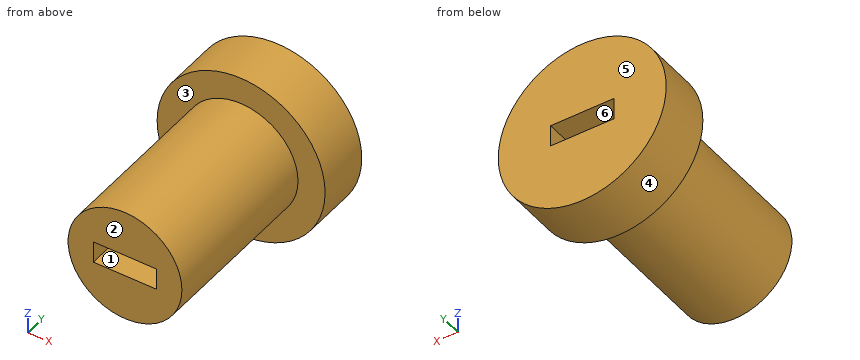
from build123d import *

# Parameters (mm, degrees)
F0_R     = 4.65
F0_R_2   = 3.15
F0_W     = 3.5
F0_H     = 1.2
F1_DEPTH = 2
F2_DEPTH = 3
F3_DEPTH = 12.5


with BuildPart() as f1:
    # F0 (on Front) → F1 (new body)
    with BuildSketch(Plane.XZ):
        Circle(F0_R)
        Circle(F0_R_2, mode=Mode.SUBTRACT)
        Circle(F0_R_2)
        Rectangle(F0_W, F0_H, mode=Mode.SUBTRACT)
    extrude(amount=F1_DEPTH)

    # F0 (on Front) → F2 (join)
    with BuildSketch(Plane.XZ):
        Circle(F0_R)
        Circle(F0_R_2, mode=Mode.SUBTRACT)
        Circle(F0_R_2)
        Rectangle(F0_W, F0_H, mode=Mode.SUBTRACT)
    extrude(amount=F2_DEPTH)

    # F0 (on Front) → F3 (join)
    with BuildSketch(Plane.XZ):
        Circle(F0_R_2)
        Rectangle(F0_W, F0_H, mode=Mode.SUBTRACT)
    extrude(amount=F3_DEPTH)


solid = f1.part
Here's how the part is built. I have some questions about the finished solid (model axes, mm). Face numbers are marked on the shaded views. A direction names the side the tool comes from. Coordinates: 2 decimals unless noted, no trailing zeros. Order: outer loops, then holes, each group sorted by start corner. A loop starts at its lowest first (then second) coordinate and runs counter-clockwise, first axis right, second up. Notation, with made-up numbers: (-3.5, -33.75) - (55.5, -33.75) arc R19 cw to (55.5, -18.75) - close; hole circle Ø1 at (31, 58). An arc over 180 degrees is marked (long way). Use CSV: the item, a comma, the result in double quotes. Start each with the question number.
1. Please list where these lines run through material, in increasing order: line 1 (Z direction, x = 0, y = -7.75); line 2 (X direction, y = -6, z = -0.5); line 3 (Z direction, x = -1.5, y = -2.75). Write a range as from..to.
2. For the marked faces 1, 2 and 3, which set-ups out of +Z, -Z, +X, -X, +Y, -Y let a thin tool reach every point of the face, with its end or its side?
3. If we mould it in two halves opening along X, with no side actions, what happens to the marked faces 4, 5 and 6? For each: +X half, -X half, draft (parallel to the pull), parting line (faces both ways), or undercut.
4. Suppose I cut it at D-D on z = -1. List the corners of the cut face in (x, y) for me, then the cut area to 3 significant figures.
5. Suppose I cut it at B-B on x = 0. List the corners of the cut face in (y, z) for me.
6. Suppose I cut it at A-A on z = 0. List the corners of the cut face in (x, y) for me, then the cut area to 3 significant figures.
7. Suppose I cut it at C-C on y = -10.25. List the corners of the cut face in (x, z) for me, then the cut area to 3 significant figures.
8. I'm going to push flat-ended pins straight in: pin 1 (5 mm diameter, centred on x = 1.5, y = -11, fed in from -Z); pin 2 (1.5 mm diameter, centred on x = -0.5, y = -8, fed in from +Z); pin 3 (1 mm diameter, centred on y = -7, z = 0, fed in from -X). Where does each tip first touch, or does it pass through?
Output:
1,line 1,"z = -3.15..-0.6, 0.6..3.15"
1,line 2,"x = -3.11..-1.75, 1.75..3.11"
1,line 3,"z = -4.4..-0.6, 0.6..4.4"
2,face 1,"+Y, -Y"
2,face 2,"+Z, -Z, +X, -X, -Y"
2,face 3,"-Y"
3,face 4,"parting line"
3,face 5,"draft"
3,face 6,"undercut"
4,outline,"(-4.54, -3) - (-2.99, -3) - (-2.99, -12.5) - (2.99, -12.5) - (2.99, -3) - (4.54, -3) - (4.54, 0) - (-4.54, 0) - close"
4,area,"84.0 mm2"
5,outline,"(-12.5, -3.15) - (-3, -3.15) - (-3, -4.65) - (0, -4.65) - (0, -0.6) - (-12.5, -0.6) - close; (-12.5, 0.6) - (0, 0.6) - (0, 4.65) - (-3, 4.65) - (-3, 3.15) - (-12.5, 3.15) - close"
6,outline,"(-4.65, -3) - (-3.15, -3) - (-3.15, -12.5) - (-1.75, -12.5) - (-1.75, 0) - (-4.65, 0) - close; (1.75, -12.5) - (3.15, -12.5) - (3.15, -3) - (4.65, -3) - (4.65, 0) - (1.75, 0) - close"
6,area,"44.0 mm2"
7,outline,"circle Ø6.3 at (0, 0); hole (-1.75, -0.6) - (1.75, -0.6) - (1.75, 0.6) - (-1.75, 0.6) - close"
7,area,"27.0 mm2"
8,pin 1,"stops at z = -3.15"
8,pin 2,"stops at z = 3.15"
8,pin 3,"stops at x = -3.15"
